from build123d import *

# Parameters (mm, degrees)
F0_R            = 9.525
F1_DEPTH        = 3.175
F2_SIZE         = 0.635
F6_ANGLE_BACK   = 22.5
F6_ANGLE        = 45
F6_COPIES_COUNT = 4
F7_SIZE         = 1.27
F8_SIZE         = 1.27


# Not quite as in the source:
# - a pattern or mirror of a feature is missing from the dataset's text; its kind, count and spacing are read off the source's solid


with BuildPart() as f1:
    # F0 (on Top) → F1 (new body)
    with BuildSketch(Plane.XY):
        Circle(F0_R)
    extrude(amount=F1_DEPTH)

    # F2
    f2_edges = [f1.edges().sort_by_distance(p)[0] for p in [
        (-9.525, 0, 3.175),
    ]]
    chamfer(f2_edges, length=F2_SIZE)

    # F3 (on Front) → F4 (revolve)
    with BuildSketch(Plane.XZ):
        Polygon((-5.08, 22.225), (-7.62, 3.175), (0, 3.175), (0, 22.225), (0, 25.4), (-5.715, 25.4), (-5.715, 28.575), (-8.255, 28.575), (-8.255, 22.225), align=None)
    revolve(axis=Axis((0, 0, 12.7), (0, 0, 1)))

    # F5 (on Right) → F6 (revolve, cut)
    with BuildSketch(Plane.YZ, mode=Mode.PRIVATE) as f6_sk:
        Polygon((-5.715, 25.4), (-5.715, 28.575), (-8.255, 28.575), (-8.255, 25.3708213568), align=None)
    f6 = revolve(f6_sk.sketch.rotate(Axis((0, 0, 12.7), (0, 0, -1)), -F6_ANGLE_BACK), axis=Axis((0, 0, 12.7), (0, 0, -1)), revolution_arc=F6_ANGLE, mode=Mode.SUBTRACT)

    # F6_copies: F6 ×4 about axis
    f6_copies_axis = Axis((0, 0, 0), (0, 0, 1))
    for i in range(1, F6_COPIES_COUNT):
        add(f6.rotate(f6_copies_axis, i * 360 / F6_COPIES_COUNT), mode=Mode.SUBTRACT)

    # F7
    f7_edges = [f1.edges().sort_by_distance(p)[0] for p in [
        (8.255, 0, 22.225),
    ]]
    chamfer(f7_edges, length=F7_SIZE)

    # F8
    f8_edges = [f1.edges().sort_by_distance(p)[0] for p in [
        (-4.041115, -4.041115, 28.575),
        (-4.041115, 4.041115, 28.575),
        (4.041115, -4.041115, 28.575),
        (4.041115, 4.041115, 28.575),
    ]]
    chamfer(f8_edges, length=F8_SIZE)


solid = f1.part
Here's how the part is built. I have some questions about the finished solid (model axes, mm). A direction names the side the tool comes from. Coordinates: 2 decimals unless noted, no trailing zeros. Loops run counter-clockwise (first coordinate to the right, second up) from the corner with the lowest first, then second, coordinate; pieces in that order, holes last.
1. Imagine slicing it at A-A, the plane z = 26.75. Please give me the cut outline in (x, y) (3 decimals), and give its area (3 significant figures).
2. Imagine slicing it at D-D, the plane z = 10. Please give me the cut outline in (x, y).
3. If we mould it in two halves opening along X, with no side actions, what happens to faces 6 (the flat face through (-2.68, -6.47, 27)), 7 (the cylindrical face through (4.06, 4.02, 26.37)), 8 (the conical face through (5.053, 3.875, 12.567)), 9 (the flat face through (-5.2, 5.3, 28.575))? For each: pulls with the +X half, pulls with the -X half, needs draft (parallel to the pull), parting line crosses it, or undercut.
4. For P1, Ø2, axis at y = -5, z = 11, coming from the +X side; P2, Ø3, axis at y = 1, z = 16.5, coming from the -X side; P3, Ø5, axis at x = -1, z = 10, coming from the -Y side, each with a flat end and sliding along its axis, tell me the tip position at first contact or that it passes through.
5. Imagine slicing it at B-B, the plane x = 0. Please give me the cut outline in (y, z) (3 decimals), and give its area (3 significant figures).
6. For faces 1 (the conical face through (0.04, -6.68, 25.39)), 2 (the conical face through (-4.41, 4.36, 27.79)), 3 (the flat face through (-6.47, 2.68, 27)), 4 (the flat face through (5, 2, 22.225)), 5 (the flat face through (5.3, 5.3, 28.575)), which set-ups out of +Z, -Z, +X, -X, +Y, -Y let a thin tool reach every point of the face, with its end or its side?
7. I need wall thicknesses on L1, parallel to Y at x = 0.25, z = 24.25; L2, parallel to Z at x = -3.25, y = 8 (3 decimals); L3, parallel to Z at x = 3, y = 1. Which ranges of each line are inside material? Lowest first, please.
Taken from the geometry:
1. outline: (-7.627, -3.159) arc R8.255 ccw to (-3.159, -7.627) - (-2.187, -5.28) arc R5.715 cw to (-5.28, -2.187) - close; (-7.627, 3.159) - (-5.28, 2.187) arc R5.715 cw to (-2.187, 5.28) - (-3.159, 7.627) arc R8.255 ccw to start; (2.187, -5.28) - (3.159, -7.627) arc R8.255 ccw to (7.627, -3.159) - (5.28, -2.187) arc R5.715 cw to start; (2.187, 5.28) arc R5.715 cw to (5.28, 2.187) - (7.627, 3.159) arc R8.255 ccw to (3.159, 7.627) - close
1. area: 55.7 mm2
2. outline: circle Ø13.42 at (0, 0)
3. face 6: undercut
3. face 7: undercut
3. face 8: parting line crosses it
3. face 9: needs draft
4. P1: stops at x = 5.24
4. P2: stops at x = -6.01
4. P3: stops at y = -7.02
5. outline: (-9.525, 0) - (9.525, 0) - (9.525, 2.54) - (8.89, 3.175) - (7.62, 3.175) - (5.08, 22.225) - (6.985, 22.225) - (8.255, 23.495) - (8.255, 25.371) - (5.715, 25.4) - (-5.715, 25.4) - (-8.255, 25.371) - (-8.255, 23.495) - (-6.985, 22.225) - (-5.08, 22.225) - (-7.62, 3.175) - (-8.89, 3.175) - (-9.525, 2.54) - close
5. area: 353 mm2
6. face 1: +Z, -Y
6. face 2: +Z
6. face 3: +Z, -X
6. face 4: none
6. face 5: +Z, +X, -X, +Y, -Y
7. L1: y = -8.25 to 8.25
7. L2: z = 0 to 3.175
7. L3: z = 0 to 25.4
